Read the model definition and answer for the solid it produces. Units are mm, in the model's axes. Face numbers are marked on the shaded views. Coordinates: 2 decimals unless noted, no trailing zeros. Write each loop counter-clockwise with the first axis right and the second up, starting at its lowest first coordinate (ties: lowest second). Pieces come first, ordered by that corner, then holes. Notation, with made-up numbers: (67.25, -40) -> (72.25, -40) arc R11 ccw to (72.25, -32) -> close; hole circle Ø3 at (30, 89.5). An arc over 180 degrees is marked (long way). Return JSON: item names as keys, results as strings.
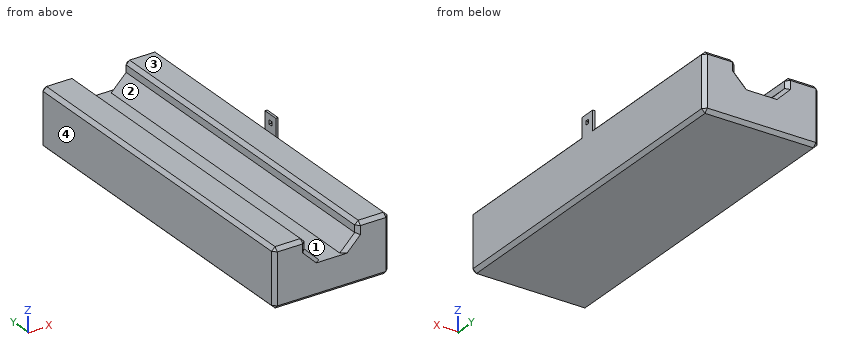
from build123d import *

# Parameters (mm, degrees)
SKETCH1_W                = 50
SKETCH1_H                = 150
BOSS_EXTRUDE1_DEPTH      = 25
CUT_EXTRUDE1_DEPTH       = 161.078105936
CHAMFER1_SIZE            = 1.5
BOSS_EXTRUDE2_DEPTH      = 7
BOSS_EXTRUDE2_DEPTH_BACK = 10
SKETCH3_W                = 1
SKETCH3_H                = 7
SKETCH4_W                = 1.8
SKETCH4_H                = 1.8
CUT_EXTRUDE2_DEPTH       = 7


with BuildPart() as part:
    # Sketch1 → Boss-Extrude1 (new body)
    with BuildSketch(Plane.XY):
        with Locations((25, 75)):
            Rectangle(SKETCH1_W, SKETCH1_H)
    extrude(amount=BOSS_EXTRUDE1_DEPTH)

    # Sketch2 → Cut-Extrude1 (cut, through all)
    with BuildSketch(Plane.XZ):
        Polygon((29.556349186, 36), (20.443650814, 36), (14, 29.556349186), (14, 20.443650814), (20.443650814, 14), (29.556349186, 14), (36, 20.443650814), (36, 29.556349186), align=None)
    extrude(amount=-CUT_EXTRUDE1_DEPTH, mode=Mode.SUBTRACT)

    # Chamfer1
    chamfer1_edges = [part.edges().sort_by_distance(p)[0] for p in [
        (50, 75, 25),
        (43, 150, 25),
        (43, 0, 25),
        (7, 150, 25),
        (14, 75, 25),
        (36, 75, 25),
        (36, 150, 22.721825407),
        (14, 150, 22.721825407),
        (36, 0, 22.721825407),
        (14, 0, 22.721825407),
        (17.221825407, 0, 17.221825407),
        (32.778174593, 0, 17.221825407),
        (32.778174593, 150, 17.221825407),
        (17.221825407, 150, 17.221825407),
        (0, 75, 25),
        (25, 150, 0),
        (50, 75, 0),
        (25, 0, 0),
        (0, 75, 0),
        (7, 0, 25),
        (0, 150, 12.5),
        (50, 150, 12.5),
        (50, 0, 12.5),
        (0, 0, 12.5),
    ]]
    chamfer(chamfer1_edges, length=CHAMFER1_SIZE)

    # Sketch3 → Boss-Extrude2 (add, two sides: drawn at the far end of the back side and taken through both)
    with BuildSketch(Plane.XY.offset(25).offset(-BOSS_EXTRUDE2_DEPTH_BACK)):
        with Locations((49.5, 75)):
            Rectangle(SKETCH3_W, SKETCH3_H)
    extrude(amount=BOSS_EXTRUDE2_DEPTH + BOSS_EXTRUDE2_DEPTH_BACK)

    # Sketch4 → Cut-Extrude2 (cut)
    with BuildSketch(Plane(origin=(50, 0, 0), x_dir=(0, 0, -1), z_dir=(1, 0, 0))):
        with Locations((-28.6, 75)):
            Rectangle(SKETCH4_W, SKETCH4_H)
    extrude(amount=-CUT_EXTRUDE2_DEPTH, mode=Mode.SUBTRACT)


solid = part.part
1. The part is cut by section D-D (x = 34). Determine the outline of the cut face in (y, z), then the cut area to 3 significant figures.
Taken from the geometry:
{"outline": "(0, 1.5) -> (1.5, 0) -> (148.5, 0) -> (150, 1.5) -> (150, 16.32) -> (148.5, 18.44) -> (1.5, 18.44) -> (0, 16.32) -> close", "area": "2,760 mm2"}
2. The part is cut by section B-B (z = 16.5). Determine the outline of the cut face in (x, y).
Taken from the geometry:
{"outline": "(0, 1.5) -> (1.5, 0) -> (15.82, 0) -> (17.94, 1.5) -> (17.94, 148.5) -> (15.82, 150) -> (1.5, 150) -> (0, 148.5) -> close; (32.06, 1.5) -> (34.18, 0) -> (48.5, 0) -> (50, 1.5) -> (50, 148.5) -> (48.5, 150) -> (34.18, 150) -> (32.06, 148.5) -> close"}
3. Flat-ended cylindrical pins translate along their axes: pin 1 Ø3.5 at (x, y) = (5.5, 110.5) entering from +Z; pin 2 Ø0.5 at (x, z) = (49.5, 28) entering from +Y; pin 3 Ø3.5 at (y, z) = (74.5, 27.5) entering from -X. Find the tip coordinate at first contact, or state that the pin passes through.
Taken from the geometry:
{"pin 1": "stops at z = 25", "pin 2": "stops at y = 78.5", "pin 3": "stops at x = 49"}
4. The part is cut by section A-A (x = 40). Determine the outline of the cut face in (y, z), then the cut area to 3 significant figures.
Taken from the geometry:
{"outline": "(0, 1.5) -> (1.5, 0) -> (148.5, 0) -> (150, 1.5) -> (150, 23.5) -> (148.5, 25) -> (1.5, 25) -> (0, 23.5) -> close", "area": "3,750 mm2"}
5. The part is cut by section C-C (y = 101). Determine the outline of the cut face in (x, z).
Taken from the geometry:
{"outline": "(0, 1.5) -> (1.5, 0) -> (48.5, 0) -> (50, 1.5) -> (50, 23.5) -> (48.5, 25) -> (37.5, 25) -> (36, 23.5) -> (36, 20.44) -> (29.56, 14) -> (20.44, 14) -> (14, 20.44) -> (14, 23.5) -> (12.5, 25) -> (1.5, 25) -> (0, 23.5) -> close"}
6. Consider L1, parallel to Z at x = 38, y = 89.5; L2, parallel to X at y = 78.5, z = 18; L3, parallel to X at y = 23, z = 24. Determine where each line is inside the solid, lowest interval first.
Taken from the geometry:
{"L1": "z = 0 to 25", "L2": "x = 0 to 16.44, 33.56 to 50", "L3": "x = 0.5 to 13.5, 36.5 to 49.5"}
7. For a pull along X with two mould halves and no side action, classify the marked faces 1, 2, 3 and 4 as +X half, -X half, draft (parallel to the pull), parting line (faces both ways), or undercut.
Taken from the geometry:
{"face 1": "undercut", "face 2": "undercut", "face 3": "draft", "face 4": "-X half"}
